For this review, take the finished solid that the model builds, in its own axes (mm). Face numbers are marked on the shaded views. A direction names the side the tool comes from. Coordinates: 2 decimals unless noted, no trailing zeros. Loops run counter-clockwise (first coordinate to the right, second up) from the corner with the lowest first, then second, coordinate; pieces in that order, holes last.
1. Clearance check with flat-ended pins moving along their axes: P1, Ø3.5, axis at y = -12.56, z = -7.25, coming from the -X side; P2, Ø1.8, axis at y = 12.56, z = -7.25, coming from the +X side; P3, Ø5, axis at y = -10.5, z = 4.5, coming from the +X side; P4, Ø1.1, axis at y = 4.5, z = -1, coming from the +X side. State where each tip first meets the part, or that it passes through.
2. To check wall thickness, follow probe 1 along X at (y, z) = (4, 2); probe 2 along X at (y, z) = (-1.5, -2); probe 3 along Y at (x, z) = (49, -7). State the ranges of each line that lie inside material, in increasing order.
3. Take a section at C-C, the plane x = 16. State the section outline as (y, z) points, then the cut area to 3 significant figures.
4. Machinability: for the marked faces 1, 2 and 3, which of the approach directions +Z, -Z, +X, -X, +Y, -Y give a long, thin tool a straight path to every point of the face, cutting with its end or side? Answer none if there is none.
5. Take a section at A-A, the plane z = 10. State the section outline as (x, y) points, then the cut area to 3 significant figures.
6. Take a section at B-B, the plane y = -8.5. State the section outline as (x, z) points, then the cut area to 3 significant figures.
7. Take a section at D-D, the plane z = -5. State the section outline as (x, y) points, then the cut area to 3 significant figures.
```python
from build123d import *

# Parameters (mm, degrees)
SKETCH2_R           = 2
BOSS_EXTRUDE1_DEPTH = 2
FILLET3_R           = 2
SKETCH3_R           = 6
BOSS_EXTRUDE2_DEPTH = 6
SKETCH4_R           = 3
BOSS_EXTRUDE3_DEPTH = 15.5
CUT_EXTRUDE1_START  = -12
CUT_EXTRUDE1_DEPTH  = 12
SKETCH6_R           = 1.5
CUT_EXTRUDE2_DEPTH  = 5
SKETCH7_R           = 1.5
CUT_EXTRUDE3_DEPTH  = 5
SKETCH9_R           = 0.5
BOSS_EXTRUDE4_DEPTH = 4
FILLET4_R           = 0.5


with BuildPart() as part:
    # Sketch1 → Revolve1 (revolve)
    with BuildSketch(Plane(origin=(0, 0, 0), x_dir=(1, 0, 0), z_dir=(0, 1, 0)), mode=Mode.PRIVATE) as revolve1_sk:
        Polygon((52, 18.5), (52, 0), (0, 0), (0, 16), (30, 16), (30, 18.5), align=None)
    revolve(revolve1_sk.sketch.rotate(Axis((0, 0, 0), (1, 0, 0)), 180), axis=Axis((0, 0, 0), (1, 0, 0)))

    # Sketch2 → Boss-Extrude1 (add)
    with BuildSketch(Plane.ZY):
        Circle(SKETCH2_R)
    extrude(amount=BOSS_EXTRUDE1_DEPTH)

    # Fillet3
    fillet3_edges = [part.edges().sort_by_distance(p)[0] for p in [
        (-2, 0, -2),
    ]]
    fillet(fillet3_edges, radius=FILLET3_R - 0.0001)  # a hair under: the kernel refuses the full size

    # Sketch3 → Boss-Extrude2 (add)
    with BuildSketch(Plane(origin=(52, 0, 0), x_dir=(0, 0, -1), z_dir=(1, 0, 0))):
        with Locations((0, 7)):
            Circle(SKETCH3_R)
    extrude(amount=BOSS_EXTRUDE2_DEPTH)

    # Sketch4 → Boss-Extrude3 (add)
    with BuildSketch(Plane(origin=(58, 0, 0), x_dir=(0, 0, -1), z_dir=(1, 0, 0))):
        with Locations((0, 7)):
            Circle(SKETCH4_R)
    extrude(amount=BOSS_EXTRUDE3_DEPTH)

    # Sketch5 → Cut-Extrude1 (cut)
    with BuildSketch(Plane(origin=(73.5, 0, 0), x_dir=(0, 0, -1), z_dir=(1, 0, 0)).offset(CUT_EXTRUDE1_START)):
        with BuildLine():
            ThreePointArc((-2.236067977, 5), (-1.224744871, 4.261387212), (0, 4))
            Line((0, 4), (0, 5))
            Line((0, 5), (-2.236067977, 5))
        make_face()
        with BuildLine():
            Line((0, 5), (0, 4))
            ThreePointArc((0, 4), (1.224744871, 4.261387212), (2.236067977, 5))
            Line((2.236067977, 5), (0, 5))
        make_face()
    extrude(amount=CUT_EXTRUDE1_DEPTH, mode=Mode.SUBTRACT)

    # Sketch6 → Cut-Extrude2 (cut)
    with BuildSketch(Plane(origin=(52, 0, 0), x_dir=(0, 0, -1), z_dir=(1, 0, 0))):
        with Locations((-14.5, 0)):
            Circle(SKETCH6_R)
        with Locations((7.25, 12.557368355)):
            Circle(SKETCH6_R)
        with Locations((7.25, -12.557368355)):
            Circle(SKETCH6_R)
    extrude(amount=-CUT_EXTRUDE2_DEPTH, mode=Mode.SUBTRACT)

    # Sketch7 → Cut-Extrude3 (cut)
    with BuildSketch(Plane(origin=(52, 0, 0), x_dir=(0, 0, -1), z_dir=(1, 0, 0))):
        with Locations((14.5, 0)):
            Circle(SKETCH7_R)
    extrude(amount=-CUT_EXTRUDE3_DEPTH, mode=Mode.SUBTRACT)

    # Sketch9 → Boss-Extrude4 (add)
    with BuildSketch(Plane.ZY):
        with Locations((0, 14)):
            Circle(SKETCH9_R)
        with Locations((0, -14)):
            Circle(SKETCH9_R)
    extrude(amount=BOSS_EXTRUDE4_DEPTH)

    # Fillet4
    fillet4_edges = [part.edges().sort_by_distance(p)[0] for p in [
        (-4, 14, -0.5),
        (-4, -14, -0.5),
    ]]
    fillet(fillet4_edges, radius=FILLET4_R)


solid = part.part
```
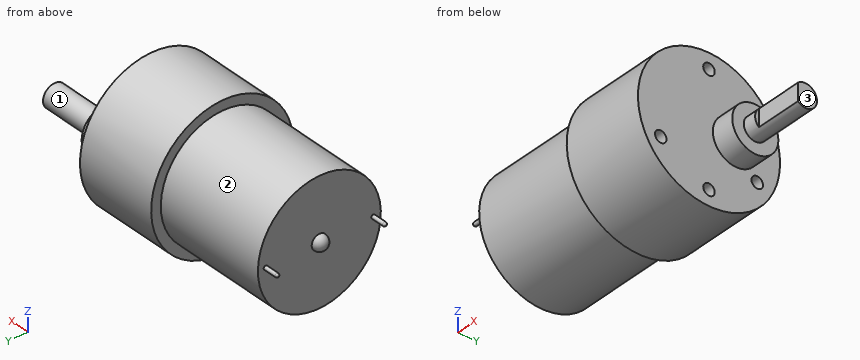
Results list:
1. P1: stops at x = 0
1. P2: stops at x = 47
1. P3: stops at x = 52
1. P4: stops at x = 73.5
2. probe 1: x = 0 to 58
2. probe 2: x = 0 to 52
2. probe 3: y = -17.12 to -14.04, -11.08 to 11.08, 14.04 to 17.12
3. outline: circle Ø32 at (0, 0)
3. area: 804 mm2
4. face 1: +X
4. face 2: -X
4. face 3: +Z, -Z, +X, +Y, -Y
5. outline: (0, -12.49) - (30, -12.49) - (30, -15.56) - (52, -15.56) - (52, 15.56) - (30, 15.56) - (30, 12.49) - (0, 12.49) - close
5. area: 1,430 mm2
6. outline: (0, -13.56) - (30, -13.56) - (30, -16.43) - (52, -16.43) - (52, 16.43) - (30, 16.43) - (30, 13.56) - (0, 13.56) - close
6. area: 1,540 mm2
7. outline: (0, -15.2) - (30, -15.2) - (30, -17.81) - (52, -17.81) - (52, 3.68) - (58, 3.68) - (58, 10.32) - (52, 10.32) - (52, 17.81) - (30, 17.81) - (30, 15.2) - (0, 15.2) - close
7. area: 1,740 mm2
